Part print with two shaded views. Sizes in mm from the minimum x, y, z corner. A direction names the side the tool comes from. Coordinates: 2 decimals unless noted, no trailing zeros. Loops run counter-clockwise (first coordinate to the right, second up) from the corner with the lowest first, then second, coordinate; pieces in that order, holes last. Notation, with made-up numbers: (-26, 43.5) -> (31, 43.5) arc R30 cw to (31, 73.5) -> close; hole circle Ø3 at (24.25, 14.5). An arc over 180 degrees is marked (long way). Use one line per item in the form item = value.
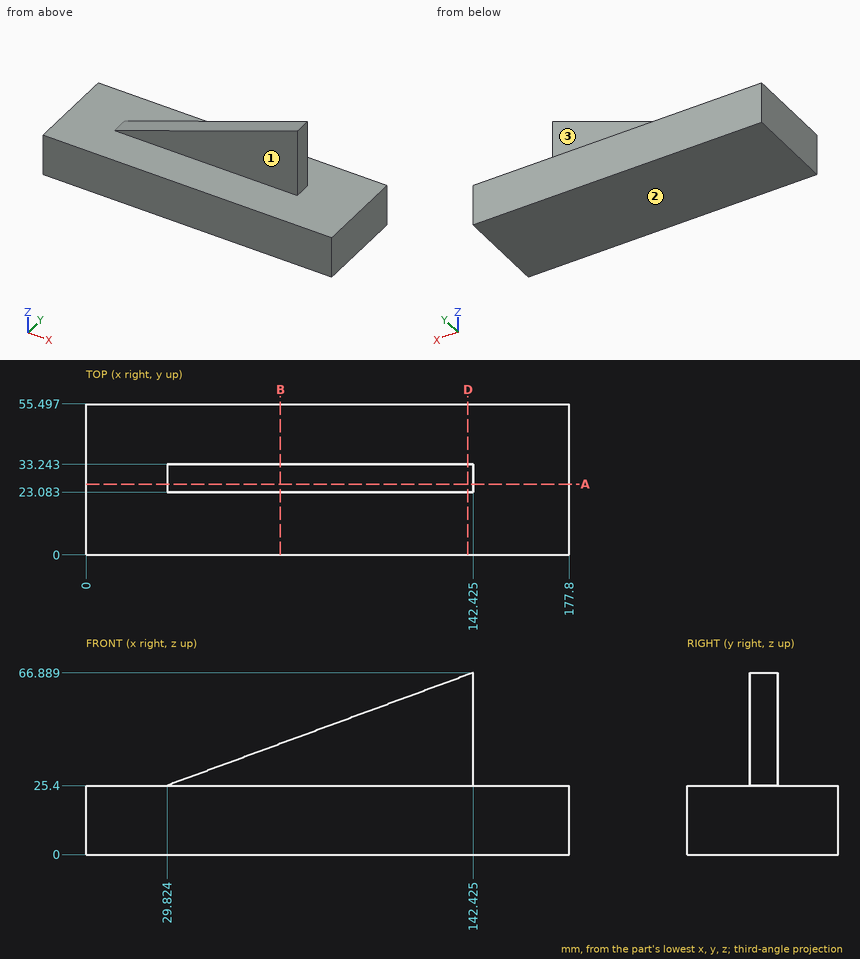
Q1. Band-saw the part on B-B, the plane x = 71.5. Write the cut outline in (y, z).
Result:
outline = (0, 0) -> (55.5, 0) -> (55.5, 25.4) -> (33.24, 25.4) -> (33.24, 40.76) -> (23.08, 40.76) -> (23.08, 25.4) -> (0, 25.4) -> close
Q2. Band-saw the part on D-D, the plane x = 140.5. Write the cut outline in (y, z).
Result:
outline = (0, 0) -> (55.5, 0) -> (55.5, 25.4) -> (33.24, 25.4) -> (33.24, 66.18) -> (23.08, 66.18) -> (23.08, 25.4) -> (0, 25.4) -> close
Q3. Band-saw the part on A-A, the plane y = 26. Write the cut outline in (x, z) (1 decimal).
Result:
outline = (0, 0) -> (177.8, 0) -> (177.8, 25.4) -> (142.4, 25.4) -> (142.4, 66.9) -> (29.8, 25.4) -> (0, 25.4) -> close
Q4. Wall check: line 1 along Y through (x, z) = (126, 57); line 2 along Z through (x, y) = (165.5, 45.5); line 3 along Z through (x, y) = (42, 23.5). Give the ranges that are in metal, low to high.
Result:
line_1 = 23.08 to 33.24
line_2 = 0 to 25.4
line_3 = 0 to 29.89
Q5. Pin check, flat tips, straight feed: pin 1 Ø8 at (y, z) = (30.5, 54.5) entering from +X (1 decimal); pin 2 Ø12.5 at (x, z) = (86.5, 43.5) entering from -Y; pin 3 Ø10 at (x, y) = (124, 22) entering from +Z. Stop position of each tip, or through.
Result:
pin_1 = 142.4
pin_2 = 23.08
pin_3 = 61.9
Q6. Which spindle directions (+Z, -Z, +X, -X, +Y, -Y) get a long thin tool onto all of the face, cutting with end or side? Do the marked faces 1, 2 and 3. Say none if no direction does.
Result:
face_1 = +Z, +X, -X, -Y
face_2 = -Z, +X, -X, +Y, -Y
face_3 = +Z, +X, -X, +Y
